Read the model definition and answer for the solid it produces. Units are mm, in the model's axes. Face numbers are marked on the shaded views. A direction names the side the tool comes from. Coordinates: 2 decimals unless noted, no trailing zeros. Write each loop counter-clockwise with the first axis right and the second up, starting at its lowest first coordinate (ties: lowest second). Pieces come first, ordered by that corner, then holes. Notation, with made-up numbers: (-27, 17) - (16, 17) arc R18 cw to (16, 35) - close; hole circle Ø2 at (52, -28). An arc over 180 degrees is marked (long way). Return JSON: item names as keys, results as strings.
```python
from build123d import *

# Parameters (mm, degrees)
SKETCH1_W           = 101
SKETCH1_H           = 95.2
BOSS_EXTRUDE1_DEPTH = 19
SHELL1_T            = -3
SKETCH3_R           = 5
BOSS_EXTRUDE2_DEPTH = 4
SKETCH4_R           = 1.6
CUT_EXTRUDE2_DEPTH  = 22
SKETCH6_W           = 28.5
SKETCH6_H           = 5.3
CUT_EXTRUDE3_DEPTH  = 22
SKETCH2_R           = 3.5
SKETCH2_R_2         = 4.5
SKETCH2_R_3         = 6.5
SKETCH2_R_4         = 2.5
SKETCH2_W           = 81
SKETCH2_H           = 53
CUT_EXTRUDE5_DEPTH  = 3


with BuildPart() as part:
    # Sketch1 → Boss-Extrude1 (new body)
    with BuildSketch(Plane(origin=(0, 0, 0), x_dir=(1, 0, 0), z_dir=(0, 1, 0))):
        with Locations((-43.75, 40.85)):
            Rectangle(SKETCH1_W, SKETCH1_H)
    extrude(amount=BOSS_EXTRUDE1_DEPTH)

    # Shell1
    shell1_openings = [part.faces().sort_by_distance(p)[0] for p in [
        (-43.75, 0, -40.85),
    ]]
    offset(amount=SHELL1_T, openings=shell1_openings, kind=Kind.INTERSECTION)

    # Sketch3 → Boss-Extrude2 (add)
    with BuildSketch(Plane.XZ.offset(-16)):
        with Locations((1.25, -82.95)):
            Circle(SKETCH3_R)
        with Locations((-88.75, -82.95)):
            Circle(SKETCH3_R)
        with Locations((-88.75, -17.95)):
            Circle(SKETCH3_R)
        with Locations((1.25, -17.95)):
            Circle(SKETCH3_R)
    extrude(amount=BOSS_EXTRUDE2_DEPTH)

    # Sketch4 → Cut-Extrude2 (cut)
    with BuildSketch(Plane.XZ.offset(-12)):
        with Locations(Location((0.25, -16.95, 0), (0, 0, 270))):
            Circle(SKETCH4_R)
        with Locations(Location((-87.75, -16.95, 0), (0, 0, 270))):
            Circle(SKETCH4_R)
        with Locations(Location((-87.75, -81.95, 0), (0, 0, 270))):
            Circle(SKETCH4_R)
        with Locations(Location((0.25, -81.95, 0), (0, 0, 270))):
            Circle(SKETCH4_R)
    extrude(amount=-CUT_EXTRUDE2_DEPTH, mode=Mode.SUBTRACT)

    # Sketch6 → Cut-Extrude3 (cut)
    with BuildSketch(Plane.ZY.offset(94.25)):
        with Locations((-49.2, 2.65)):
            Rectangle(SKETCH6_W, SKETCH6_H)
    extrude(amount=-CUT_EXTRUDE3_DEPTH, mode=Mode.SUBTRACT)

    # Sketch2 → Cut-Extrude5 (cut)
    with BuildSketch(Plane(origin=(0, 19, 0), x_dir=(1, 0, 0), z_dir=(0, 1, 0))):
        with Locations(Location((-87.75, 81.95, 0), (0, 0, 270))):
            Circle(SKETCH2_R)
        with Locations(Location((0.25, 81.95, 0), (0, 0, 270))):
            Circle(SKETCH2_R)
        with Locations(Location((-87.75, 16.95, 0), (0, 0, 270))):
            Circle(SKETCH2_R)
        with Locations(Location((0.25, 16.95, 0), (0, 0, 270))):
            Circle(SKETCH2_R)
        with Locations(Location((-6.25, 5.95, 0), (0, 0, 270))):
            Circle(SKETCH2_R_2)
        with Locations(Location((-24.95, 5.75, 0), (0, 0, 270))):
            Circle(SKETCH2_R_3)
        with Locations(Location((-39.95, 5.55, 0), (0, 0, 270))):
            Circle(SKETCH2_R_4)
        with Locations((-43.6, 49.95)):
            Rectangle(SKETCH2_W, SKETCH2_H)
    extrude(amount=-CUT_EXTRUDE5_DEPTH, mode=Mode.SUBTRACT)


solid = part.part
```
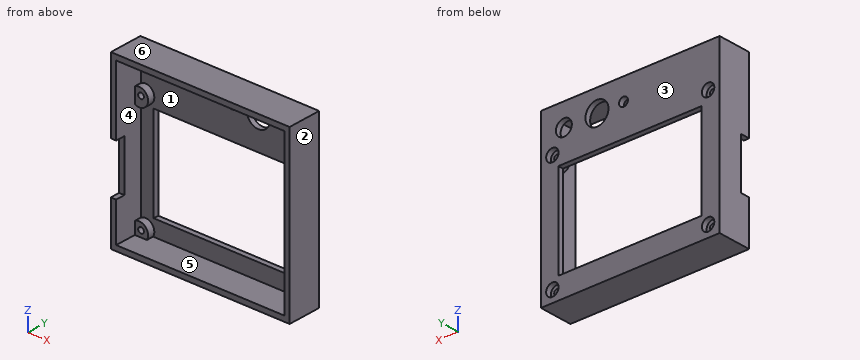
(1) A cutting plane is placed at A-A (x = -69.5). Determine the outline of the cut face in (y, z), and give its area (3 significant figures).
Answer:
{"outline": "(0, -88.45) - (19, -88.45) - (19, -76.45) - (16, -76.45) - (16, -85.45) - (0, -85.45) - close; (0, 3.75) - (16, 3.75) - (16, -23.45) - (19, -23.45) - (19, 6.75) - (0, 6.75) - close", "area": "223 mm²"}
(2) A cutting plane is placed at B-B (z = -27). Determine the outline of the cut face in (x, y).
Answer:
{"outline": "(-94.25, 0) - (-91.25, 0) - (-91.25, 16) - (-84.1, 16) - (-84.1, 19) - (-94.25, 19) - close; (-3.1, 16) - (3.75, 16) - (3.75, 0) - (6.75, 0) - (6.75, 19) - (-3.1, 19) - close"}
(3) Straight lines are drawn through the part: line 1 (X direction, y = 17.2, z = -16.95); line 2 (X direction, y = 17.4, z = -5.75); line 3 (Z direction, x = -79, y = 2). For each, find the intervals that lie inside material, in ascending order. Write a range as from..to.
Answer:
{"line 1": "-94.25..-91.25, -84.25..-3.25, 3.75..6.75", "line 2": "-94.25..-42.44, -37.46..-31.45, -18.45..-10.75, -1.75..6.75", "line 3": "-88.45..-85.45, 3.75..6.75"}
(4) Flat-ended cylindrical pins translate along their axes: P1, Ø4, axis at x = -87.75, z = -16.95, coming from the -Y side; P2, Ø0.9, axis at x = -92.5, z = -51, coming from the -Y side; P3, Ø9, axis at x = 0.25, z = -81.95, coming from the +Y side; P4, Ø1.9, axis at x = -87.75, z = -81.95, coming from the +Y side. Find the tip coordinate at first contact, or state that the pin passes through.
Answer:
{"P1": "y = 12", "P2": "y = 5.3", "P3": "y = 19", "P4": "through"}
(5) A cutting plane is placed at D-D (z = -5.95). Determine the outline of the cut face in (x, y), and give its area (3 significant figures).
Answer:
{"outline": "(-94.25, 0) - (-91.25, 0) - (-91.25, 16) - (-42.42, 16) - (-42.42, 19) - (-94.25, 19) - close; (-37.48, 16) - (-31.45, 16) - (-31.45, 19) - (-37.48, 19) - close; (-18.45, 16) - (-10.75, 16) - (-10.75, 19) - (-18.45, 19) - close; (-1.75, 16) - (3.75, 16) - (3.75, 0) - (6.75, 0) - (6.75, 19) - (-1.75, 19) - close", "area": "318 mm²"}
(6) Determine the mould class of the marked faces 3, 4, 5 and 6 for opening direction Z: +Z half, -Z half, draft (parallel to the pull), parting line (faces both ways), or undercut.
Answer:
{"face 3": "draft", "face 4": "undercut", "face 5": "undercut", "face 6": "+Z half"}
(7) A cutting plane is placed at C-C (x = -23). Determine the outline of the cut face in (y, z), and give its area (3 significant figures).
Answer:
{"outline": "(0, -88.45) - (19, -88.45) - (19, -76.45) - (16, -76.45) - (16, -85.45) - (0, -85.45) - close; (0, 3.75) - (16, 3.75) - (16, 0.45) - (19, 0.45) - (19, 6.75) - (0, 6.75) - close; (16, -23.45) - (19, -23.45) - (19, -11.95) - (16, -11.95) - close", "area": "185 mm²"}
(8) Which of the six approach directions +Z, -Z, +X, -X, +Y, -Y give full straight-line access (tool end or side, diameter ignored) to the marked faces 1 and 2?
Answer:
{"face 1": "-Y", "face 2": "+Z, -Z, +X, +Y, -Y"}
